Source: CAD feature listing. Evaluate the final solid. Frame: model axes, mm. Face numbers are marked on the shaded views. A direction names the side the tool comes from. Give positions to 0.01 mm unless a question says otherwise; leave off trailing zeros. Loops run counter-clockwise (first coordinate to the right, second up) from the corner with the lowest first, then second, coordinate; pieces in that order, holes last.
Autodesk Inventor part; units mm, degrees
ref_plane "YZ Plane" through (0, 0, 0) normal (1, 0, 0) x (0, 1, 0)
ref_plane "XZ Plane" through (0, 0, 0) normal (0, 1, 0) x (-1, 0, 0)
ref_plane "XY Plane" through (0, 0, 0) normal (0, 0, 1) x (1, 0, 0)
sketch "Sketch1" plane through (0, 0, 0) normal (0, 0, 1) x (1, 0, 0)
  arc A0 (0, 31.75) -> (21.1582, 52.9082) centre (0, 52.9082) ccw
  line L0 (0, 31.75) -> (38.8128, 31.75) construction
  line L1 (30.6832, 0) -> (30.6832, 86.3474)
  line L2 (21.1582, 52.9082) -> (21.1582, 86.3474)
  line L3 (21.1582, 86.3474) -> (30.6832, 86.3474)
  line L4 (0, 79.9974) -> (0, 0) construction
  line L5 (0, 31.75) -> (0, 0)
  line L6 (30.6832, 0) -> (0, 0)
  dimension "pipeDiameter" = 42.3164
  dimension "d1" = 31.75
  dimension "width" = 9.525
revolve "Revolution1" add sketch "Sketch1" angle 360 about axis through (30.6832, 0, 0) along (-1, 0, 0)
sketch "Sketch2" plane through (30.6832, 0, 0) normal (1, 0, 0) x (0, 0, -1)
  line L0 (-3.9595, 6.858) -> (3.9595, 6.858)
  line L1 (3.9595, 6.858) -> (7.9189, 0)
  line L2 (7.9189, 0) -> (3.9595, -6.858)
  line L3 (3.9595, -6.858) -> (-3.9595, -6.858)
  line L4 (-3.9595, -6.858) -> (-7.9189, 0)
  line L5 (-7.9189, 0) -> (-3.9595, 6.858)
  point P0 (0, 0)
  point P1 (0, 0)
  dimension "hexWidth" = 13.716
extrude "Extrusion1" cut sketch "Sketch2" against normal through all
sketch "Sketch3" plane through (30.6832, 0, 0) normal (1, 0, 0) x (0, 0, -1)
  point P0 (0, 0)
  point P1 (-25.4, 0)
  point P2 (-12.7, -21.997)
  point P3 (12.7, -21.997)
  point P4 (25.4, 0)
  point P5 (12.7, 21.997)
  point P6 (-12.7, 21.997)
  dimension "d7" = 25.4
  dimension "d10" = 360
hole "Hole1" at (30.6832, 0, 25.4) at (30.6832, -21.997, 12.7) at (30.6832, -21.997, -12.7) at (30.6832, 0, -25.4) at (30.6832, 21.997, -12.7) at (30.6832, 21.997, 12.7) direction (-1, 0, 0) diameter 6.7564 end through all counterbore diameter 13.97 counterbore depth 4.7752
properties part number "halfWheelForHangingAndMovingV2"
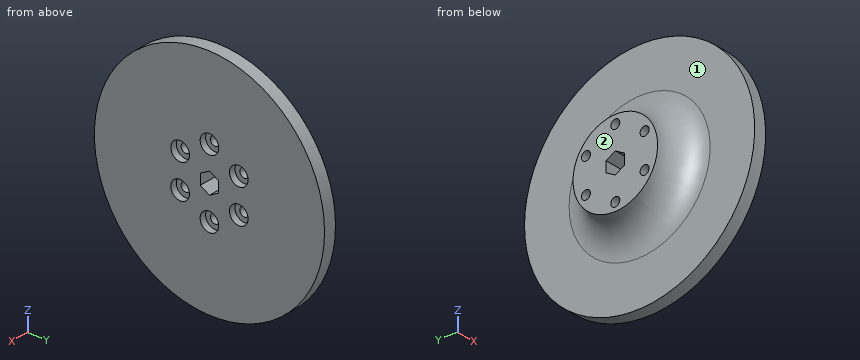
1) Contact query for flat-ended pins moving along their axis: P1, Ø3, axis at x = 20.5, y = 35, coming from the +Z side; P2, Ø7, axis at y = -22.5, z = 12.5, coming from the +X side; P3, Ø6, axis at y = 0, z = 25.4, coming from the +X side; P4, Ø3, axis at y = 27, z = -58.5, coming from the -X side. Output: stop coordinate, or through.
Checks:
P1: stops at z = 79.52
P2: stops at x = 25.91
P3: passes through
P4: stops at x = 21.16
2) Cut plane C-C (x = 12.5). Return loops of the section in (y, z), and give its area (3 significant figures).
Checks:
outline: circle Ø71.67 at (0, 0); hole circle Ø6.76 at (-22, -12.7); hole circle Ø6.76 at (-22, 12.7); hole (-6.86, -3.96) - (0, -7.92) - (6.86, -3.96) - (6.86, 3.96) - (0, 7.92) - (-6.86, 3.96) - close; hole circle Ø6.76 at (0, -25.4); hole circle Ø6.76 at (0, 25.4); hole circle Ø6.76 at (22, -12.7); hole circle Ø6.76 at (22, 12.7)
area: 3,660 mm2
3) Ray query, probe 1 along Z at (x, y) = (11, -25); probe 2 along Y at (x, z) = (6, 13.5); probe 3 along Z at (x, y) = (16, 0). Return the intervals inside material, ascending.
Checks:
probe 1: z = -24.26 to -14.25, -11.15 to 11.15, 14.25 to 24.26
probe 2: y = -29.69 to -25.28, -18.71 to 18.71, 25.28 to 29.69
probe 3: z = -39.06 to -28.78, -22.02 to -7.92, 7.92 to 22.02, 28.78 to 39.06
4) Cut plane A-A (z = 0). Return loops of the section in (x, y).
Checks:
outline: (0, -31.75) arc R21.16 cw to (21.16, -52.91) - (21.16, -86.35) - (30.68, -86.35) - (30.68, -6.86) - (0, -6.86) - close; (0, 6.86) - (30.68, 6.86) - (30.68, 86.35) - (21.16, 86.35) - (21.16, 52.91) arc R21.16 cw to (0, 31.75) - close
5) Reachability of the marked faces 1 and 2 from +Z, -Z, +X, -X, +Y, -Y: full face, straight path, thin tool, end or side. Return the list, or none.
Checks:
face 1: -X
face 2: +Z, -Z, -X, +Y, -Y
6) Cut plane B-B (x = 28.5). Return loops of the section in (y, z) (1 decimal), and give its area (3 significant figures).
Checks:
outline: circle Ø172.7 at (0, 0); hole circle Ø14 at (-22, -12.7); hole circle Ø14 at (-22, 12.7); hole circle Ø14 at (0, -25.4); hole circle Ø14 at (0, 25.4); hole (-6.9, -4) - (0, -7.9) - (6.9, -4) - (6.9, 4) - (0, 7.9) - (-6.9, 4) - close; hole circle Ø14 at (22, -12.7); hole circle Ø14 at (22, 12.7)
area: 22,300 mm2
7) Cut plane D-D (y = 60). Return loops of the section in (x, z), and give its area (3 significant figures).
Checks:
outline: (21.16, -62.1) - (30.68, -62.1) - (30.68, 62.1) - (21.16, 62.1) - close
area: 1,180 mm2
